```python
from build123d import *

# Parameters (mm, degrees)
SKETCH2_R          = 5
CUT_EXTRUDE1_DEPTH = 4
CUT_EXTRUDE2_START = 4
SKETCH3_R          = 2
CUT_EXTRUDE2_DEPTH = 6.5
CUT_EXTRUDE4_START = -9
SKETCH4_R          = 2.5
CUT_EXTRUDE4_DEPTH = 6.5


with BuildPart() as part:
    # Sketch1 → Revolve1 (revolve)
    with BuildSketch(Plane.XY, mode=Mode.PRIVATE) as revolve1_sk:
        Polygon((-1.5, 15), (-1.5, 12.25), (1.5, 12.25), (1.5, 15), (6.5, 15), (6.5, 0), (-6.5, 0), (-6.5, 15), align=None)
    revolve(revolve1_sk.sketch.rotate(Axis((6.5, 0, 0), (-1, 0, 0)), 90), axis=Axis((6.5, 0, 0), (-1, 0, 0)))

    # Sketch2 → Cut-Extrude1 (cut)
    with BuildSketch(Plane(origin=(6.5, 0, 0), x_dir=(0, 0, -1), z_dir=(1, 0, 0))):
        Circle(SKETCH2_R)
    extrude(amount=-CUT_EXTRUDE1_DEPTH, mode=Mode.SUBTRACT)

    # Sketch3 → Cut-Extrude2 (cut)
    with BuildSketch(Plane(origin=(2.5, 0, 0), x_dir=(0, 0, -1), z_dir=(1, 0, 0)).offset(CUT_EXTRUDE2_START)):
        Circle(SKETCH3_R)
    extrude(amount=-CUT_EXTRUDE2_DEPTH, mode=Mode.SUBTRACT)

    # Sketch4 → Cut-Extrude4 (cut)
    with BuildSketch(Plane(origin=(2.5, 0, 0), x_dir=(0, 0, -1), z_dir=(1, 0, 0)).offset(CUT_EXTRUDE4_START)):
        with Locations(Location((0, 0, 0), (0, 0, 180))):
            Circle(SKETCH4_R)
    extrude(amount=CUT_EXTRUDE4_DEPTH, mode=Mode.SUBTRACT)


solid = part.part
```
Input: part model. Units: mm. Frame: model coordinates. A direction names the side the tool comes from. Give positions to 0.01 mm unless a question says otherwise; leave off trailing zeros. Write each loop counter-clockwise with the first axis right and the second up, starting at its lowest first coordinate (ties: lowest second). Pieces come first, ordered by that corner, then holes. Notation, with made-up numbers: (55, 37) - (62, 37) arc R17 cw to (62, 43) - close; hole circle Ø8 at (66, 28.5). An arc over 180 degrees is marked (long way). Write item = value, one per line. Start each with the question number.
1. Mould query, pull axis X, two halves, no side actions, for faces 1 (the flat face through (2.5, -2.2, 0.1)), 2 (the cylindrical face through (-3.96, -12.65, -8.06)), 3 (the flat face through (-1.5, 11, 6)). Classes: released by +X, released by -X, zero draft, split by the parting line, or undercut.
2. Ray query, L1, parallel to Y at x = 1.85, z = 0; L2, parallel to Y at x = 4.2, z = 0; L3, parallel to X at y = -2.25, z = -13. Return the intervals inside material, ascending.
3. Access query for faces 4 (the cylindrical face through (0.021, -3.68, -11.684)), 5 (the flat face through (0, -2, -1)), 6 (the cylindrical face through (4.53, -4.88, 1.08)), 7 (the cylindrical face through (1, -2, 0)). Directions: +Z, -Z, +X, -X, +Y, -Y. A direction counts if a zero-diameter tool reaches every point of the face in a straight line with its end or side. Return the directions, or none.
4. Section query C-C, the plane x = 0.75. Output: boundary loops of the cut face in (y, z).
5. First-contact query: pin 1 Ø1 at (x, z) = (-2, -11) entering from -Y; pin 2 Ø3 at (y, z) = (0, 0) entering from -X; pin 3 Ø6 at (x, z) = (2, -8.5) entering from +Y; pin 4 Ø5 at (y, z) = (0, 0) entering from +X. Flat tips, straight axial feed; report the tip coordinate or a pass-through.
6. Section query D-D, the plane z = -5.75. Output: boundary loops of the cut face in (x, y).
7. Section query A-A, the plane z = 0. Output: boundary loops of the cut face in (x, y).
Check sheet entries:
q1.face_1 = released by +X
q1.face_2 = zero draft
q1.face_3 = undercut
q2.L1 = -15 to -2, 2 to 15
q2.L2 = -15 to -5, 5 to 15
q2.L3 = -6.5 to -1.5, 1.5 to 6.5
q3.face_4 = none
q3.face_5 = -X
q3.face_6 = +X
q3.face_7 = +X, -X
q4.outline = circle Ø24.5 at (0, 0); hole circle Ø4 at (0, 0)
q5.pin_1 = -10.71
q5.pin_2 = through
q5.pin_3 = 13.96
q5.pin_4 = 2.5
q6.outline = (-6.5, -13.85) - (-1.5, -13.85) - (-1.5, -10.82) - (1.5, -10.82) - (1.5, -13.85) - (6.5, -13.85) - (6.5, 13.85) - (1.5, 13.85) - (1.5, 10.82) - (-1.5, 10.82) - (-1.5, 13.85) - (-6.5, 13.85) - close
q7.outline = (-6.5, -15) - (-1.5, -15) - (-1.5, -12.25) - (1.5, -12.25) - (1.5, -15) - (6.5, -15) - (6.5, -5) - (2.5, -5) - (2.5, -2) - (0, -2) - (0, -2.5) - (-6.5, -2.5) - close; (-6.5, 2.5) - (0, 2.5) - (0, 2) - (2.5, 2) - (2.5, 5) - (6.5, 5) - (6.5, 15) - (1.5, 15) - (1.5, 12.25) - (-1.5, 12.25) - (-1.5, 15) - (-6.5, 15) - close
